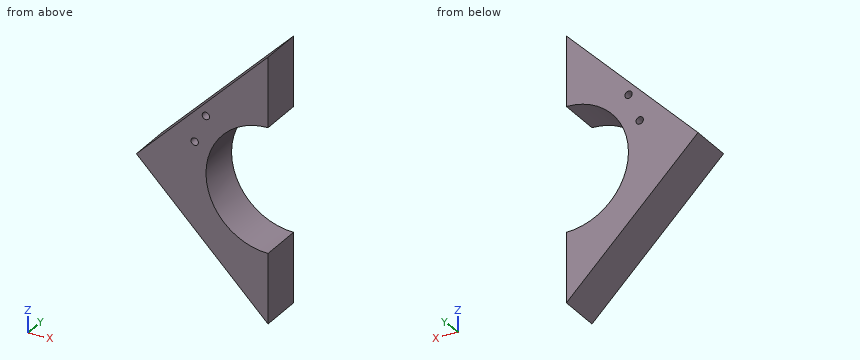
from build123d import *

# Parameters (mm, degrees)
SKETCH1_R           = 3
BOSS_EXTRUDE1_DEPTH = 36


with BuildPart() as part:
    # Sketch1 → Boss-Extrude1 (new body)
    with BuildSketch(Plane(origin=(0, 0, 0), x_dir=(1, 0, 0), z_dir=(0, 1, 0))):
        with BuildLine():
            Line((0, 0), (-107.763073453, 107.763073453))
            Line((-107.763073453, 107.763073453), (0, 215.526146906))
            Line((0, 215.526146906), (0, 158.563073453))
            ThreePointArc((0, 158.563073453), (-50.8, 107.763073453), (0, 56.963073453))
            Line((0, 56.963073453), (0, 0))
        make_face()
        with Locations(Location((-60.033365723, 84.782103064, 0), (0, 0, 270))):
            Circle(SKETCH1_R, mode=Mode.SUBTRACT)
        with Locations(Location((-50.902581789, 61.509183506, 0), (0, 0, 270))):
            Circle(SKETCH1_R, mode=Mode.SUBTRACT)
    extrude(amount=BOSS_EXTRUDE1_DEPTH)


solid = part.part
Here's how the part is built. I have some questions about the finished solid (model axes, mm). Coordinates: 2 decimals unless noted, no trailing zeros. Write each loop counter-clockwise with the first axis right and the second up, starting at its lowest first coordinate (ties: lowest second). Pieces come first, ordered by that corner, then holes.
Item 1: I want a section at A-A on x = -20. Write out the boundary of the cut face in (y, z).
Item 2: I want a section at C-C on z = -67.5. Write out the boundary of the cut face in (x, y).
Item 3: Will these pins go through, and if not, where does the flat tip stop? pin 1 (1.5 mm diameter, centred on x = -63.5, y = 26, fed in from +Z); pin 2 (2 mm diameter, centred on y = 19, z = -89, fed in from -X); pin 3 (3 mm diameter, centred on x = -23, y = 17, fed in from -Z); pin 4 (12 mm diameter, centred on x = -69, z = -155.5, fed in from -Y).
Item 4: I want a section at D-D on x = -70.5. Write out the boundary of the cut face in (y, z), and give its area (3 significant figures).
Item 5: I want a section at B-B on y = 33.5. Write out the boundary of the cut face in (x, z), and give its area (3 significant figures).
Item 6: If I drill on line 1 (Z direction, x = -15, y = 32.5); line 2 (Z direction, x = -41, y = 12); line 3 (X direction, y = 11, z = -84), over which ranges is the centre line in solid material (lowest first)?
Findings below:
1. outline: (0, -195.53) - (36, -195.53) - (36, -154.46) - (0, -154.46) - close; (0, -61.07) - (36, -61.07) - (36, -20) - (0, -20) - close
2. outline: (-67.5, 0) - (-30.98, 0) - (-30.98, 36) - (-67.5, 36) - close
3. pin 1: stops at z = -62.75
3. pin 2: stops at x = -90
3. pin 3: stops at z = -194.03
3. pin 4: passes through
4. outline: (0, -145.03) - (36, -145.03) - (36, -70.5) - (0, -70.5) - close
4. area: 2,680 mm2
5. outline: (-107.76, -107.76) - (0, -215.53) - (0, -158.56) arc R50.8 cw to (0, -56.96) - (0, 0) - close; hole circle Ø6 at (-60.03, -84.78); hole circle Ø6 at (-50.9, -61.51)
5. area: 7,500 mm2
6. line 1: z = -200.53 to -156.3, -59.23 to -15
6. line 2: z = -174.53 to -137.76, -77.77 to -41
6. line 3: x = -84 to -62.93, -57.14 to -44.9
